Geometry check sheet. Reference: the model listing, model coordinates, mm. Face numbers are marked on the shaded views. Round coordinates to 2 decimals unless told otherwise and drop trailing zeros. Write each loop counter-clockwise with the first axis right and the second up, starting at its lowest first coordinate (ties: lowest second). Pieces come first, ordered by that corner, then holes. Notation, with made-up numbers: M 82.5,-25.75 L 131.5,-25.75 A18 ccw 131.5,-6.75 Z; hole C 88,-26 d10. An arc over 180 degrees is marked long. One line per item, written item: value. Start each with the question number.
1. Section check A-A (y = -252.5). Record the boundary of the cut face in (x, z), and give its area (3 significant figures).
2. Scan lines: probe 1 along X at (y, z) = (-78, 9); probe 2 along X at (y, z) = (-287.3, -23.65); probe 3 along Z at (x, y) = (-6, 71.5). Record each from-to range of solid material in increasing order. Write a range as [from, to].
3. Release check for a two-part mould opening along Z. For the marked faces 1, 2 and 3 record: pulls with the +Z half, pulls with the -Z half, needs draft (parallel to the pull), parting line crosses it, or undercut.
4. Depth check by flat-ended pin: P1, Ø4, axis at x = -15.7, y = 87.3, coming from the -Z side; P2, Ø12.5, axis at x = -14, y = -137.5, coming from the +Z side; P3, Ø8, axis at x = -15.7, y = -287.3, coming from the +Z side. Enter the tip coordinate at first touch or a pass-through.
5. Section check B-B (z = 16). Record the boundary of the cut face in (x, y).
6. Section check C-C (y = 70). Record the boundary of the cut face in (x, z).
from build123d import *

# Parameters (mm, degrees)
SKETCH1_W                    = 600
SKETCH1_H                    = 100
BASE_FLANGE1_DEPTH           = 1.5
SKETCHED_START               = -300
SKETCHED_BEND1_DEPTH         = 600
SKETCHED_BEND1_2_DEPTH       = 600
SKETCHED_BEND2_DEPTH         = 600
SKETCHED_BEND2_2_DEPTH       = 600
F_4_0_4_DIAMETER_HOLE1_D     = 4
F_5_0_5_DIAMETER_HOLE1_D     = 5
F_5_0_5_DIAMETER_HOLE1_DEPTH = 1.5
CUT_EXTRUDE1_REACH           = 307.656
SKETCH12_W                   = 102
SKETCH12_H                   = 16


# Read off the part's stored shape, not the designer's step: Sketched Bend1, Sketched Bend2
# Sheet-metal steps are written as plain solids
with BuildPart() as part:
    # Sketch1 → Base-Flange1 (new body)
    with BuildSketch(Plane.YZ):
        Rectangle(SKETCH1_W, SKETCH1_H)
    extrude(amount=-BASE_FLANGE1_DEPTH)

    # Sketched Bend1 outline → Sketched Bend1 (cut)
    with BuildSketch(Plane(origin=(0, 0, 0), x_dir=(1, 0, 0), z_dir=(0, 1, 0)).offset(SKETCHED_START)):
        with BuildLine():
            Line((-1.5, 50), (-1.5, 24.198076212))
            ThreePointArc((-1.5, 24.198076212), (-0.401923788, 23.1), (0, 21.6))
            Line((0, 21.6), (0, 50))
            Line((0, 50), (-1.5, 50))
        make_face()
    extrude(amount=SKETCHED_BEND1_DEPTH, mode=Mode.SUBTRACT)

    # Sketched Bend1 2 outline → Sketched Bend1 2 (add)
    with BuildSketch(Plane(origin=(0, 0, 0), x_dir=(1, 0, 0), z_dir=(0, 1, 0)).offset(SKETCHED_START)):
        with BuildLine():
            Line((-27.865708265, 24.6), (-27.865708265, 23.1))
            Line((-27.865708265, 23.1), (-3, 23.1))
            ThreePointArc((-3, 23.1), (-1.939339828, 22.660660172), (-1.5, 21.6))
            Line((-1.5, 21.6), (-1.5, 24.198076212))
            ThreePointArc((-1.5, 24.198076212), (-2.223542865, 24.497777479), (-3, 24.6))
            Line((-3, 24.6), (-27.865708265, 24.6))
        make_face()
    extrude(amount=SKETCHED_BEND1_2_DEPTH)

    # Sketched Bend2 outline → Sketched Bend2 (cut)
    with BuildSketch(Plane(origin=(0, 0, 0), x_dir=(1, 0, 0), z_dir=(0, 1, 0)).offset(SKETCHED_START)):
        with BuildLine():
            ThreePointArc((0, -22.499377385), (-0.401923789, -23.999377385), (-1.5, -25.097453597))
            Line((-1.5, -25.097453597), (-1.5, -50))
            Line((-1.5, -50), (0, -50))
            Line((0, -50), (0, -22.499377385))
        make_face()
    extrude(amount=SKETCHED_BEND2_DEPTH, mode=Mode.SUBTRACT)

    # Sketched Bend2 2 outline → Sketched Bend2 2 (add)
    with BuildSketch(Plane(origin=(0, 0, 0), x_dir=(1, 0, 0), z_dir=(0, 1, 0)).offset(SKETCHED_START)):
        with BuildLine():
            ThreePointArc((-1.5, -22.499377385), (-1.771271934, -23.35974204), (-2.486969785, -23.908916317))
            Line((-2.486969785, -23.908916317), (-25.745986918, -32.374506231))
            Line((-25.745986918, -32.374506231), (-25.232956703, -33.784045162))
            Line((-25.232956703, -33.784045162), (-1.97393957, -25.318455248))
            ThreePointArc((-1.97393957, -25.318455248), (-1.732145215, -25.218300747), (-1.5, -25.097453597))
            Line((-1.5, -25.097453597), (-1.5, -22.499377385))
        make_face()
    extrude(amount=SKETCHED_BEND2_2_DEPTH)

    # Ø4.0 (4) Diameter Hole1 (through all)
    with Locations(Plane(origin=(7.906287599, 0, 21.72234665), x_dir=(0.9396926207859094, 0, -0.34202014332566616), z_dir=(0.34202014332566616, 0, 0.9396926207859094))):
        with Locations((-23.21431814, 287.3), (-23.21431814, 12.7)):
            f_4_0_4_diameter_hole1 = Hole(F_4_0_4_DIAMETER_HOLE1_D / 2)

    # Mirror1: Ø4.0 (4) Diameter Hole1 across plane
    add(f_4_0_4_diameter_hole1.mirror(Plane.ZX), mode=Mode.SUBTRACT)

    # Ø5.0 (5) Diameter Hole1
    with Locations(Plane.YX.offset(24.6)):
        with Locations((-287.3, -15.7), (-87.3, -15.7), (87.3, -15.7), (287.3, -15.7)):
            Hole(F_5_0_5_DIAMETER_HOLE1_D / 2, depth=F_5_0_5_DIAMETER_HOLE1_DEPTH)

    # Sketch12 → Cut-Extrude1 (cut, up to next)
    with BuildSketch(Plane(origin=(7.906287599, 0, 21.72234665), x_dir=(0, -1, 0), z_dir=(0.34202014332566616, 0, 0.9396926207859094)), mode=Mode.PRIVATE) as cut_extrude1_sk1:
        with Locations((218, -27.266047183)):
            Rectangle(SKETCH12_W, SKETCH12_H)
    cut_extrude1_tool1 = extrude(cut_extrude1_sk1.sketch, amount=-CUT_EXTRUDE1_REACH, mode=Mode.PRIVATE) & part.part
    add(cut_extrude1_tool1.solids().sort_by_distance((-17.715416, -218, 31.047884))[0], mode=Mode.SUBTRACT)


solid = part.part
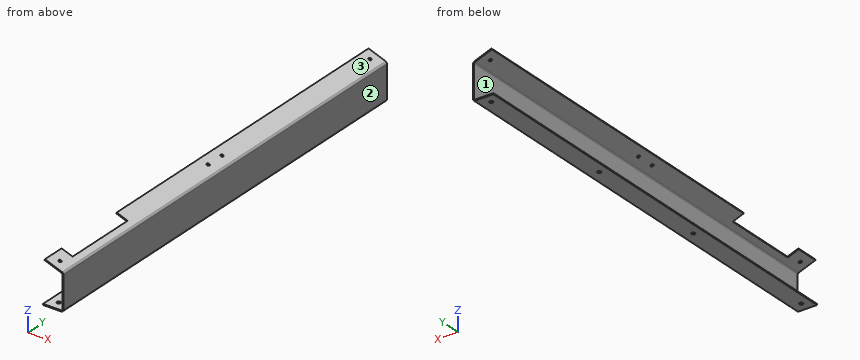
Result sheet:
1. outline: M -27.87,-24.6 L -3,-24.6 A3 ccw 0,-21.6 L 0,22.5 A3 ccw -1.97,25.32 L -10.2,28.31 L -10.71,26.9 L -2.49,23.91 A1.5 cw -1.5,22.5 L -1.5,-21.6 A1.5 cw -3,-23.1 L -27.87,-23.1 Z
1. area: 126 mm2
2. probe 1: x = [-1.5, 0]
2. probe 2: x = [-27.87, -18.2], [-13.2, -0.81]
2. probe 3: z = [-24.6, -23.1], [25.19, 26.78]
3. face 1: undercut
3. face 2: needs draft
3. face 3: pulls with the +Z half
4. P1: stops at z = 27.99
4. P2: stops at z = 31.97
4. P3: stops at z = 31.77
5. outline: M -1.5,-300 L 0,-300 L 0,300 L -1.5,300 Z
6. outline: M -27.87,-24.6 L -3,-24.6 A3 ccw 0,-21.6 L 0,22.5 A3 ccw -1.97,25.32 L -25.23,33.78 L -25.75,32.37 L -2.49,23.91 A1.5 cw -1.5,22.5 L -1.5,-21.6 A1.5 cw -3,-23.1 L -27.87,-23.1 Z
